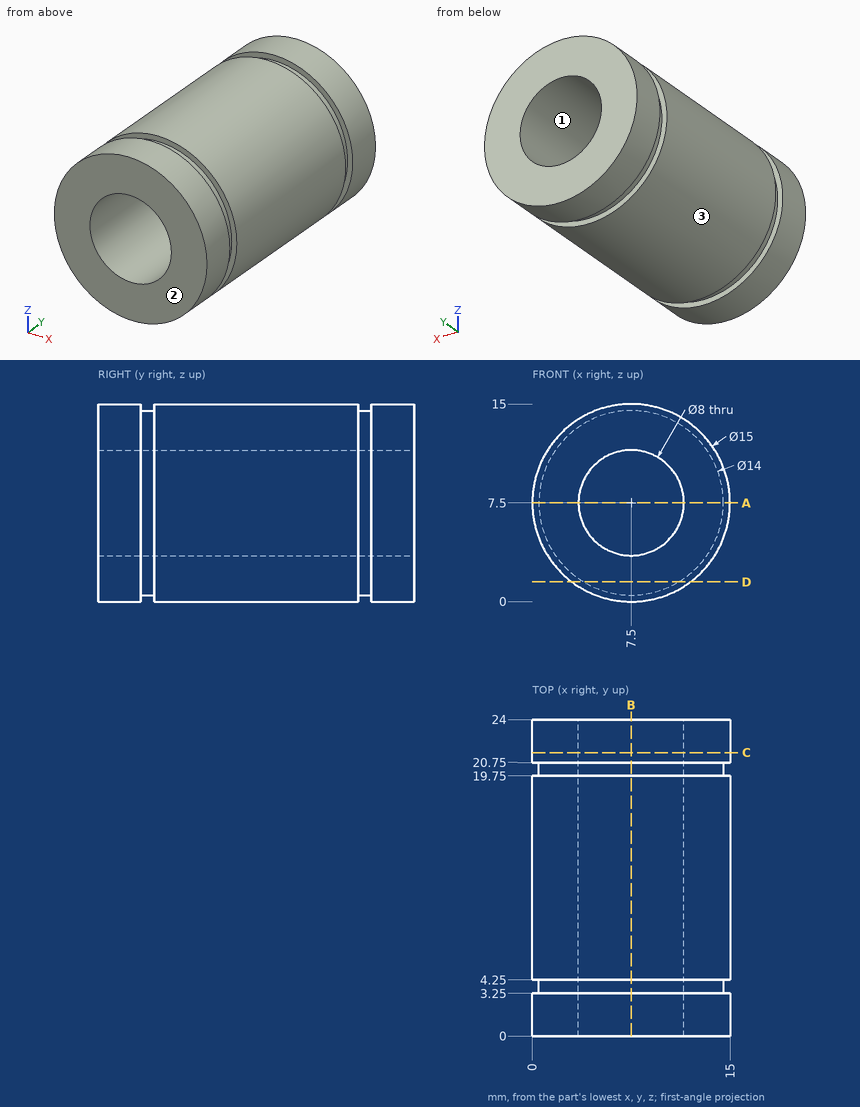
Check sheet for the drawn part. Datum: minimum x, y, z corner. Units: mm. Round coordinates to 2 decimals unless told otherwise and drop trailing zeros. Loops run counter-clockwise (first coordinate to the right, second up) from the corner with the lowest first, then second, coordinate; pieces in that order, holes last.
Item 1: Cross-section at B-B on x = 7.5. Record the boundary of the cut face in (y, z).
Item 2: Cross-section at A-A on z = 7.5. Record the boundary of the cut face in (x, y).
Item 3: Thickness scan on line 1 (Z direction, x = 7.5, y = 16); line 2 (X direction, y = 17.5, z = 9.25); line 3 (X direction, y = 3.75, z = 8.25). Record the ranges inside material, lowest first.
Item 4: Mould release check, pull along X, two halves, no side actions. Record for the marked faces 1, 2 and 3: pulls with the +X half, pulls with the -X half, needs draft (parallel to the pull), parting line crosses it, or undercut.
Item 5: Cross-section at C-C on y = 21.5. Record the boundary of the cut face in (x, z), then the cut area to 3 significant figures.
Item 6: Cross-section at D-D on z = 1.5. Record the boundary of the cut face in (x, y), then the cut area to 3 significant figures.
Item 7: Gauge pin test, flat ends, axial feed: pin 1 (1 mm diameter, centred on y = 18.5, z = 2, fed in from +X); pin 2 (1 mm diameter, centred on x = 4.5, y = 19.5, fed in from -Z); pin 3 (6 mm diameter, centred on x = 5, z = 12, fed in from -Y); pin 4 (1.5 mm diameter, centred on x = 4, y = 14.5, fed in from +Z). Record the tip position at first contact, or that the pin passes through.
Answer sheet:
1. outline: (0, 0) - (3.25, 0) - (3.25, 0.5) - (4.25, 0.5) - (4.25, 0) - (19.75, 0) - (19.75, 0.5) - (20.75, 0.5) - (20.75, 0) - (24, 0) - (24, 3.5) - (0, 3.5) - close; (0, 11.5) - (24, 11.5) - (24, 15) - (20.75, 15) - (20.75, 14.5) - (19.75, 14.5) - (19.75, 15) - (4.25, 15) - (4.25, 14.5) - (3.25, 14.5) - (3.25, 15) - (0, 15) - close
2. outline: (0, 0) - (3.5, 0) - (3.5, 24) - (0, 24) - (0, 20.75) - (0.5, 20.75) - (0.5, 19.75) - (0, 19.75) - (0, 4.25) - (0.5, 4.25) - (0.5, 3.25) - (0, 3.25) - close; (11.5, 0) - (15, 0) - (15, 3.25) - (14.5, 3.25) - (14.5, 4.25) - (15, 4.25) - (15, 19.75) - (14.5, 19.75) - (14.5, 20.75) - (15, 20.75) - (15, 24) - (11.5, 24) - close
3. line 1: z = 0 to 3.5, 11.5 to 15
3. line 2: x = 0.21 to 3.9, 11.1 to 14.79
3. line 3: x = 0.54 to 3.57, 11.43 to 14.46
4. face 1: undercut
4. face 2: needs draft
4. face 3: parting line crosses it
5. outline: circle Ø15 at (7.5, 7.5); hole circle Ø8 at (7.5, 7.5)
5. area: 126 mm2
6. outline: (3, 0) - (12, 0) - (12, 3.25) - (11.11, 3.25) - (11.11, 4.25) - (12, 4.25) - (12, 19.75) - (11.11, 19.75) - (11.11, 20.75) - (12, 20.75) - (12, 24) - (3, 24) - (3, 20.75) - (3.89, 20.75) - (3.89, 19.75) - (3, 19.75) - (3, 4.25) - (3.89, 4.25) - (3.89, 3.25) - (3, 3.25) - close
6. area: 212 mm2
7. pin 1: stops at x = 13.09
7. pin 2: stops at z = 0.43
7. pin 3: stops at y = 0
7. pin 4: stops at z = 14.48
